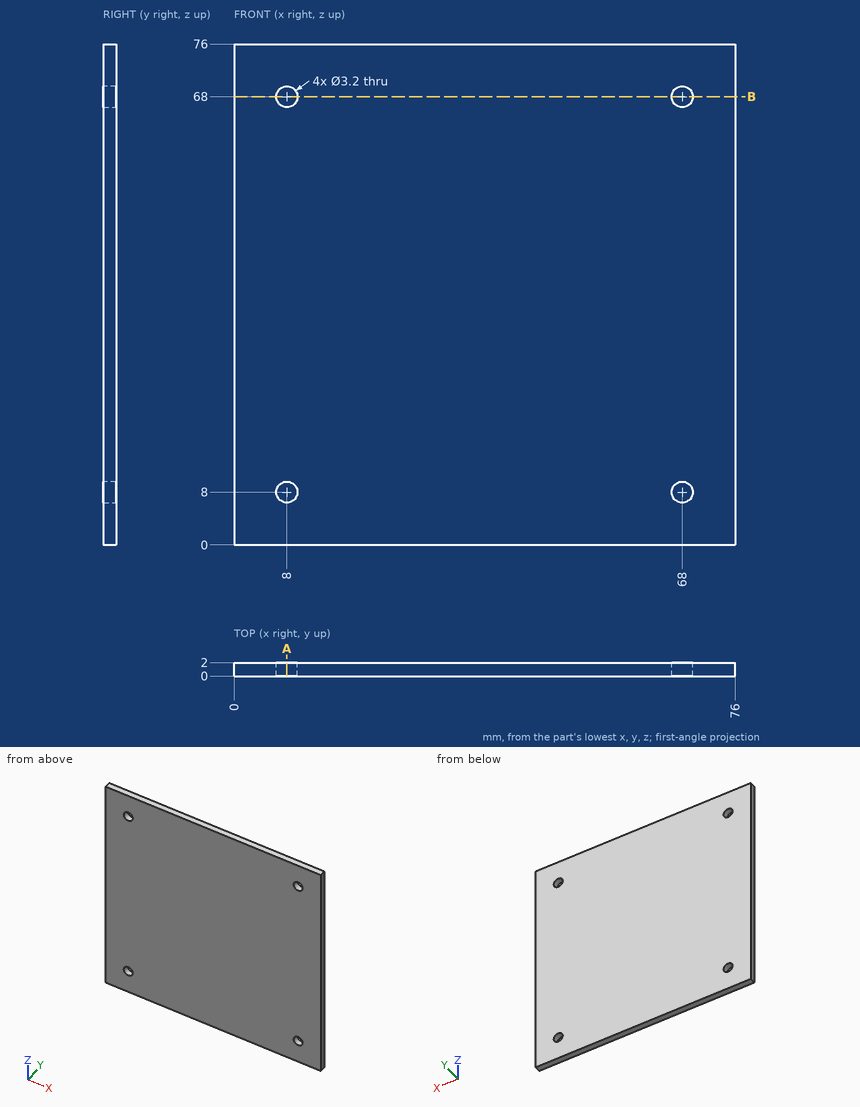
Geometry check sheet. Reference: drawing and pictorial views, mm from the part's lowest x, y, z. Coordinates: 2 decimals unless noted, no trailing zeros. Loops run counter-clockwise (first coordinate to the right, second up) from the corner with the lowest first, then second, coordinate; pieces in that order, holes last. Notation, with made-up numbers: (35, 85.25) -> (85, 85.25) arc R20 cw to (85, 103.25) -> close; hole circle Ø11 at (73.25, 26.25). An arc over 180 degrees is marked (long way). Write item = value, one per line. Start each with the question number.
1. Section check B-B on z = 68. Record the cut outline in (x, y), then the cut area to 3 significant figures.
2. Material ranges on line 1 (X direction, y = 0.75, z = 8); line 2 (Z direction, x = 8.5, y = 0.4), recorded low to high.
3. Section check A-A on x = 8. Record the cut outline in (y, z).
Responses:
q1.outline = (0, 0) -> (6.4, 0) -> (6.4, 2) -> (0, 2) -> close; (9.6, 0) -> (66.4, 0) -> (66.4, 2) -> (9.6, 2) -> close; (69.6, 0) -> (76, 0) -> (76, 2) -> (69.6, 2) -> close
q1.area = 139 mm2
q2.line_1 = 0 to 6.4, 9.6 to 66.4, 69.6 to 76
q2.line_2 = 0 to 6.48, 9.52 to 66.48, 69.52 to 76
q3.outline = (0, 0) -> (2, 0) -> (2, 6.4) -> (0, 6.4) -> close; (0, 9.6) -> (2, 9.6) -> (2, 66.4) -> (0, 66.4) -> close; (0, 69.6) -> (2, 69.6) -> (2, 76) -> (0, 76) -> close
